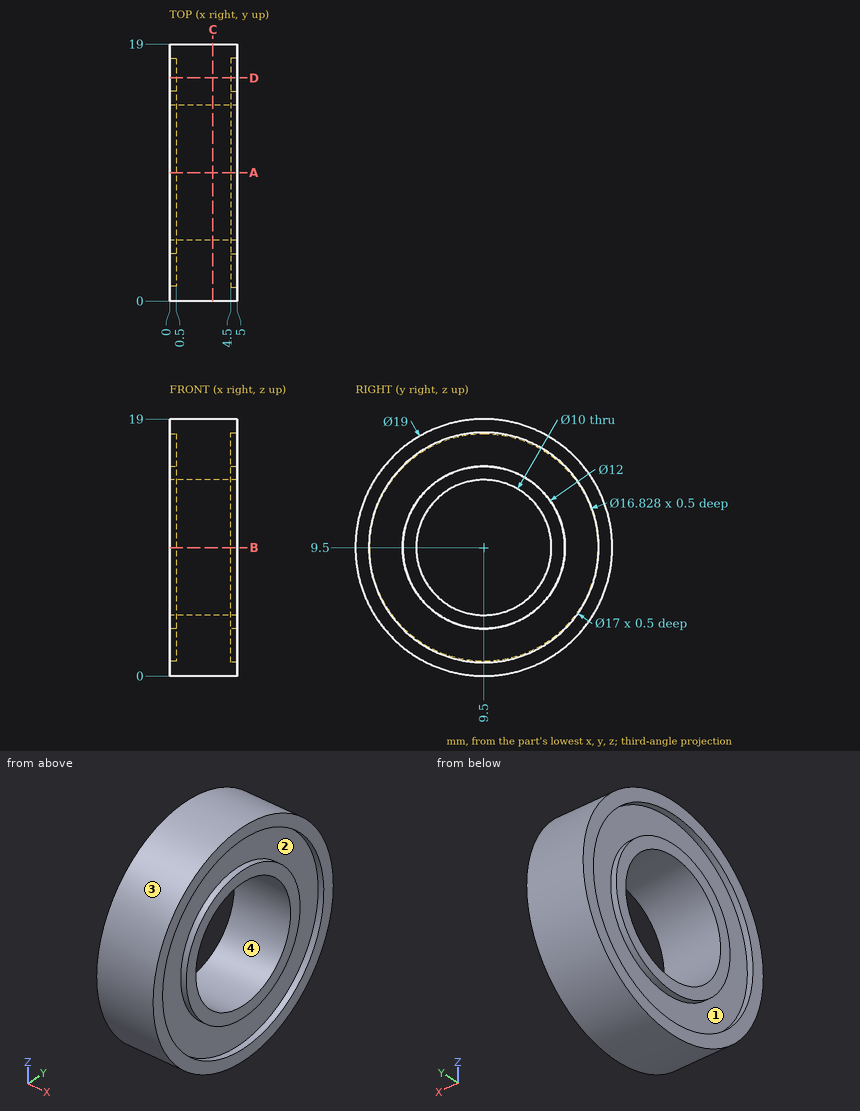
Here's the drawing with two shaded views (mm, measured from the low corner). I have some questions. A direction names the side the tool comes from. Round coordinates to 2 decimals unless told otherwise and drop trailing zeros. Loops run counter-clockwise (first coordinate to the right, second up) from the corner with the lowest first, then second, coordinate; pieces in that order, holes last.
1. Will these pins go through, and if not, where does the flat tip stop? pin 1 (3 mm diameter, centred on x = 3.5, y = 15, fed in from -Z); pin 2 (10 mm diameter, centred on y = 4, z = 4.5, fed in from -X); pin 3 (1 mm diameter, centred on y = 3, z = 10.5, fed in from +X); pin 4 (3 mm diameter, centred on x = 3.5, y = 14.5, fed in from -Z).
Answers:
pin 1: stops at z = 0.88
pin 2: stops at x = 0
pin 3: stops at x = 4.5
pin 4: stops at z = 0.67
2. For the marked faces 1 and 2, which set-ups out of +Z, -Z, +X, -X, +Y, -Y let a thin tool reach every point of the face, with its end or its side?
Answers:
face 1: -X
face 2: +X
3. Suppose I cut it at C-C, the plane x = 3.2. Please give me the cut outline in (y, z).
Answers:
outline: circle Ø19 at (9.5, 9.5); hole circle Ø10 at (9.5, 9.5)
4. Suppose I cut it at A-A, the plane y = 9.5. Please give me the cut outline in (x, z) (1 decimal).
Answers:
outline: (0, 0) - (5, 0) - (5, 1) - (4.5, 1) - (4.5, 3.5) - (5, 3.5) - (5, 4.5) - (0, 4.5) - (0, 3.5) - (0.5, 3.5) - (0.5, 1.1) - (0, 1.1) - close; (0, 14.5) - (5, 14.5) - (5, 15.5) - (4.5, 15.5) - (4.5, 18) - (5, 18) - (5, 19) - (0, 19) - (0, 17.9) - (0.5, 17.9) - (0.5, 15.5) - (0, 15.5) - close
5. Suppose I cut it at D-D, the plane y = 16.5. Please give me the cut outline in (x, z).
Answers:
outline: (0, 3.08) - (5, 3.08) - (5, 4.68) - (4.5, 4.68) - (4.5, 14.32) - (5, 14.32) - (5, 15.92) - (0, 15.92) - (0, 14.17) - (0.5, 14.17) - (0.5, 4.83) - (0, 4.83) - close
6. If I drill on probe 1 along Z at (x, y) = (2.5, 9.5); probe 2 along X at (y, z) = (7.5, 16.25); probe 3 along Y at (x, z) = (2.3, 13), over which ranges is the centre line in solid material (lowest first)?
Answers:
probe 1: z = 0 to 4.5, 14.5 to 19
probe 2: x = 0.5 to 4.5
probe 3: y = 0.67 to 5.93, 13.07 to 18.33
7. Thinking about a two-plate mould opening in Y: for the marked faces 3 and 4, which applies, released by +Y, released by -Y, zero draft, split by the parting line, or undercut?
Answers:
face 3: split by the parting line
face 4: undercut
